from build123d import *

# Parameters (mm, degrees)
SKETCH1_R                = 18.5
SKETCH1_R_2              = 16.5
BOSS_EXTRUDE1_DEPTH      = 108
SKETCH2_R                = 18.5
BOSS_EXTRUDE2_DEPTH      = 2
SKETCH3_R                = 10
CUT_EXTRUDE1_DEPTH       = 114.06856327
BOSS_EXTRUDE3_START      = -3
SKETCH4_W                = 40
SKETCH4_H                = 40
SKETCH4_R                = 18.5
BOSS_EXTRUDE3_DEPTH      = 3
FILLET1_R                = 4
CUT_EXTRUDE2_DEPTH       = 119.74342087
CIRPATTERN1_COUNT        = 2
CIRPATTERN1_ANGLE        = 90
CIRPATTERN1_COPY_1_DEPTH = 119.74342087
SKETCH6_R                = 1.05
CUT_EXTRUDE3_DEPTH       = 111.675200474
FILLET2_R                = 1
CHAMFER1_SIZE            = 0.5


with BuildPart() as part:
    # Sketch1 → Boss-Extrude1 (new body)
    with BuildSketch(Plane(origin=(0, 0, 0), x_dir=(1, 0, 0), z_dir=(0, 1, 0))):
        with Locations(Location((0, 0, 0), (0, 0, 270))):
            Circle(SKETCH1_R)
        with Locations(Location((0, 0, 0), (0, 0, 270))):
            Circle(SKETCH1_R_2, mode=Mode.SUBTRACT)
    extrude(amount=BOSS_EXTRUDE1_DEPTH)

    # Sketch2 → Boss-Extrude2 (add)
    with BuildSketch(Plane(origin=(0, 108, 0), x_dir=(1, 0, 0), z_dir=(0, 1, 0))):
        with Locations(Location((0, 0, 0), (0, 0, 270))):
            Circle(SKETCH2_R)
    extrude(amount=BOSS_EXTRUDE2_DEPTH)

    # Sketch3 → Cut-Extrude1 (cut, through all)
    with BuildSketch(Plane(origin=(0, 110, 0), x_dir=(1, 0, 0), z_dir=(0, 1, 0))):
        with Locations(Location((0, 0, 0), (0, 0, 270))):
            Circle(SKETCH3_R)
    extrude(amount=-CUT_EXTRUDE1_DEPTH, mode=Mode.SUBTRACT)

    # Sketch4 → Boss-Extrude3 (add)
    with BuildSketch(Plane(origin=(0, 110, 0), x_dir=(1, 0, 0), z_dir=(0, 1, 0)).offset(BOSS_EXTRUDE3_START)):
        Rectangle(SKETCH4_W, SKETCH4_H)
        with Locations(Location((0, 0, 0), (0, 0, 270))):
            Circle(SKETCH4_R, mode=Mode.SUBTRACT)
    extrude(amount=BOSS_EXTRUDE3_DEPTH)

    # Fillet1
    fillet1_edges = [part.edges().sort_by_distance(p)[0] for p in [
        (-20, 108.5, 20),
        (-20, 108.5, -20),
        (20, 108.5, -20),
        (20, 108.5, 20),
    ]]
    fillet(fillet1_edges, radius=FILLET1_R)

    # Sketch5 → Cut-Extrude2 (cut, through all)
    with BuildSketch(Plane.XY.offset(20)):
        Polygon((14, 110), (17, 110), (16, 109), (15, 109), align=None)
    cut_extrude2 = extrude(amount=-CUT_EXTRUDE2_DEPTH, mode=Mode.SUBTRACT)

    # Mirror1: Cut-Extrude2 across plane
    add(cut_extrude2.mirror(Plane(origin=(0, 0, 0), x_dir=(0, 0, 1), z_dir=(1, 0, 0))), mode=Mode.SUBTRACT)

    # CirPattern1: Cut-Extrude2 ×2 about axis
    cirpattern1_axis = Axis((0, 0, 0), (0, 1, 0))
    for i in range(1, CIRPATTERN1_COUNT):
        add(cut_extrude2.rotate(cirpattern1_axis, i * CIRPATTERN1_ANGLE / (CIRPATTERN1_COUNT - 1)), mode=Mode.SUBTRACT)

    # CirPattern1 copy 1 sketch → CirPattern1 copy 1 (cut, through all)
    with BuildSketch(Plane(origin=(20, 0, 0), x_dir=(0, 0, 1), z_dir=(1, 0, 0))):
        Polygon((14, -110), (17, -110), (16, -109), (15, -109), align=None)
    extrude(amount=-CIRPATTERN1_COPY_1_DEPTH, mode=Mode.SUBTRACT)

    # Sketch6 → Cut-Extrude3 (cut, through all)
    with BuildSketch(Plane.XZ.offset(-107)):
        with Locations(Location((15.5, 15.5, 0), (0, 0, 270))):
            Circle(SKETCH6_R)
        with Locations(Location((-15.5, 15.5, 0), (0, 0, 270))):
            Circle(SKETCH6_R)
        with Locations(Location((-15.5, -15.5, 0), (0, 0, 270))):
            Circle(SKETCH6_R)
        with Locations(Location((15.5, -15.5, 0), (0, 0, 270))):
            Circle(SKETCH6_R)
    extrude(amount=-CUT_EXTRUDE3_DEPTH, mode=Mode.SUBTRACT)

    # Fillet2
    fillet2_edges = [part.edges().sort_by_distance(p)[0] for p in [
        (0, 108, -10),
        (0, 107, -18.5),
    ]]
    fillet(fillet2_edges, radius=FILLET2_R)

    # Chamfer1
    chamfer1_edges = [part.edges().sort_by_distance(p)[0] for p in [
        (0, 0, -18.5),
        (0, 0, -16.5),
    ]]
    chamfer(chamfer1_edges, length=CHAMFER1_SIZE)


solid = part.part
Design review of the part built by this model. Coordinates are the model's own, in mm. A direction names the side the tool comes from. Round coordinates to 2 decimals unless told otherwise and drop trailing zeros. Write each loop counter-clockwise with the first axis right and the second up, starting at its lowest first coordinate (ties: lowest second). Pieces come first, ordered by that corner, then holes. Notation, with made-up numbers: M 67.5,-5 L 72.5,-5 A21 cw 72.5,19 Z; hole C -24.5,61 d10. An arc over 180 degrees is marked long. One line per item, written item: value. Start each with the question number.
1. Clearance check with flat-ended pins moving along their axes: P1, Ø2.5, axis at x = 15.5, z = 15.5, coming from the -Y side; P2, Ø5, axis at x = -9.5, y = 11, coming from the +Z side; P3, Ø1.3, axis at x = -15.5, z = 15.5, coming from the -Y side; P4, Ø16.5, axis at x = -1.5, z = 5.5, coming from the -Y side. State where each tip first meets the part, or that it passes through.
2. To check wall thickness, follow probe 1 along X at (y, z) = (108.1, -15.5); probe 2 along X at (y, z) = (109.3, 0). State the ranges of each line that lie inside material, in increasing order. Write a range as from..to.
3. For faces 4 (the face through (-11, 108, 3)), 5 (the face through (15.55, 108.11, -14.45)), list the 3-axis set-ups (+Z, -Z, +X, -X, +Y, -Y) from which the entire face can be reached by the end or side of a thin tool; tool diameter is ignored.
4. Draft analysis for pull direction Z (two halves, no side actions). For faces 1 (the face through (0, 108, 20)), 2 (the face through (18, 110, 18)), 3 (the face through (-15.45, 108.11, -14.45)), state which applies: pulls with the +Z half, pulls with the -Z half, needs draft (parallel to the pull), parting line crosses it, or undercut.
5. Take a section at C-C on y = 39.5. State the section outline as (x, z) points, then the cut area to 3 significant figures.
Computed:
1. P1: stops at y = 107
1. P2: stops at z = 17.12
1. P3: passes through
1. P4: stops at y = 108
2. probe 1: x = -20..-16.55, -14.45..14.45, 16.55..20
2. probe 2: x = -20..-16.3, -14.7..-10, 10..14.7, 16.3..20
3. face 4: -Y
3. face 5: +Y, -Y
4. face 1: pulls with the +Z half
4. face 2: needs draft
4. face 3: undercut
5. outline: C 0,0 d37; hole C 0,0 d33
5. area: 220 mm²
